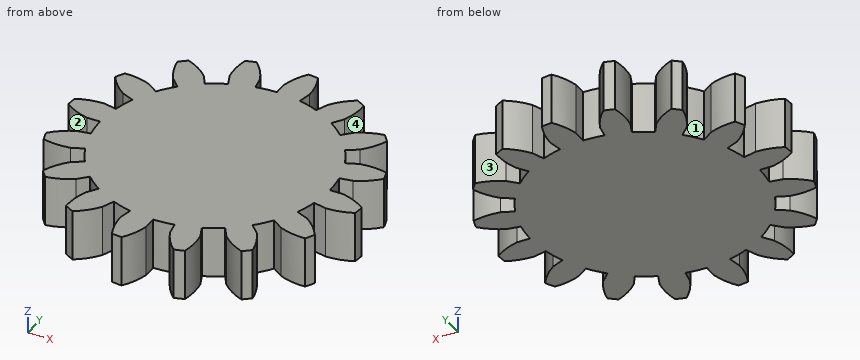
from build123d import *

# Parameters (mm, degrees)
BOSS_EXTRU_1_DEPTH           = 3
R_P_TITION_CIRCULAIRE2_COUNT = 16
ESQUISSE5_R                  = 6.75
BOSS_EXTRU_2_DEPTH           = 3


with BuildPart() as part:
    # Esquisse4 → Boss.-Extru.1 (new body)
    with BuildSketch(Plane.XY):
        with BuildLine():
            Line((0, 7.517540966), (0, 6.75))
            ThreePointArc((0, 6.75), (0.719454333, 6.711548664), (1.430711931, 6.59663273))
            Line((1.430711931, 6.59663273), (1.593397859, 7.346734339))
            ThreePointArc((1.593397859, 7.346734339), (1.508511555, 8.147299885), (1.256427196, 8.911867969))
            ThreePointArc((1.256427196, 8.911867969), (0.959272444, 8.948731551), (0.661055861, 8.975689675))
            ThreePointArc((0.661055861, 8.975689675), (0.252643326, 8.281924527), (0, 7.517540966))
        make_face()
    extrude(amount=BOSS_EXTRU_1_DEPTH)


with BuildPart() as r_p_tition_circulaire2_1:
    # R_p_tition circulaire2: pattern copy
    add(part.part.rotate(Axis((0, 0, 0), (0, 0, 1)), 1 * 360 / R_P_TITION_CIRCULAIRE2_COUNT))


with BuildPart() as r_p_tition_circulaire2_2:
    # R_p_tition circulaire2: pattern copy
    add(part.part.rotate(Axis((0, 0, 0), (0, 0, 1)), 2 * 360 / R_P_TITION_CIRCULAIRE2_COUNT))


with BuildPart() as r_p_tition_circulaire2_3:
    # R_p_tition circulaire2: pattern copy
    add(part.part.rotate(Axis((0, 0, 0), (0, 0, 1)), 3 * 360 / R_P_TITION_CIRCULAIRE2_COUNT))


with BuildPart() as r_p_tition_circulaire2_4:
    # R_p_tition circulaire2: pattern copy
    add(part.part.rotate(Axis((0, 0, 0), (0, 0, 1)), 4 * 360 / R_P_TITION_CIRCULAIRE2_COUNT))


with BuildPart() as r_p_tition_circulaire2_5:
    # R_p_tition circulaire2: pattern copy
    add(part.part.rotate(Axis((0, 0, 0), (0, 0, 1)), 5 * 360 / R_P_TITION_CIRCULAIRE2_COUNT))


with BuildPart() as r_p_tition_circulaire2_6:
    # R_p_tition circulaire2: pattern copy
    add(part.part.rotate(Axis((0, 0, 0), (0, 0, 1)), 6 * 360 / R_P_TITION_CIRCULAIRE2_COUNT))


with BuildPart() as r_p_tition_circulaire2_7:
    # R_p_tition circulaire2: pattern copy
    add(part.part.rotate(Axis((0, 0, 0), (0, 0, 1)), 7 * 360 / R_P_TITION_CIRCULAIRE2_COUNT))


with BuildPart() as r_p_tition_circulaire2_8:
    # R_p_tition circulaire2: pattern copy
    add(part.part.rotate(Axis((0, 0, 0), (0, 0, 1)), 8 * 360 / R_P_TITION_CIRCULAIRE2_COUNT))


with BuildPart() as r_p_tition_circulaire2_9:
    # R_p_tition circulaire2: pattern copy
    add(part.part.rotate(Axis((0, 0, 0), (0, 0, 1)), 9 * 360 / R_P_TITION_CIRCULAIRE2_COUNT))


with BuildPart() as r_p_tition_circulaire2_10:
    # R_p_tition circulaire2: pattern copy
    add(part.part.rotate(Axis((0, 0, 0), (0, 0, 1)), 10 * 360 / R_P_TITION_CIRCULAIRE2_COUNT))


with BuildPart() as r_p_tition_circulaire2_11:
    # R_p_tition circulaire2: pattern copy
    add(part.part.rotate(Axis((0, 0, 0), (0, 0, 1)), 11 * 360 / R_P_TITION_CIRCULAIRE2_COUNT))


with BuildPart() as r_p_tition_circulaire2_12:
    # R_p_tition circulaire2: pattern copy
    add(part.part.rotate(Axis((0, 0, 0), (0, 0, 1)), 12 * 360 / R_P_TITION_CIRCULAIRE2_COUNT))


with BuildPart() as r_p_tition_circulaire2_13:
    # R_p_tition circulaire2: pattern copy
    add(part.part.rotate(Axis((0, 0, 0), (0, 0, 1)), 13 * 360 / R_P_TITION_CIRCULAIRE2_COUNT))


with BuildPart() as r_p_tition_circulaire2_14:
    # R_p_tition circulaire2: pattern copy
    add(part.part.rotate(Axis((0, 0, 0), (0, 0, 1)), 14 * 360 / R_P_TITION_CIRCULAIRE2_COUNT))


with BuildPart() as r_p_tition_circulaire2_15:
    # R_p_tition circulaire2: pattern copy
    add(part.part.rotate(Axis((0, 0, 0), (0, 0, 1)), 15 * 360 / R_P_TITION_CIRCULAIRE2_COUNT))


with BuildPart() as part_1:
    add(part.part)

    add(r_p_tition_circulaire2_1.part)  # Boss.-Extru.2 merges R_p_tition circulaire2_1

    add(r_p_tition_circulaire2_2.part)  # Boss.-Extru.2 merges R_p_tition circulaire2_2

    add(r_p_tition_circulaire2_3.part)  # Boss.-Extru.2 merges R_p_tition circulaire2_3

    add(r_p_tition_circulaire2_4.part)  # Boss.-Extru.2 merges R_p_tition circulaire2_4

    add(r_p_tition_circulaire2_5.part)  # Boss.-Extru.2 merges R_p_tition circulaire2_5

    add(r_p_tition_circulaire2_6.part)  # Boss.-Extru.2 merges R_p_tition circulaire2_6

    add(r_p_tition_circulaire2_7.part)  # Boss.-Extru.2 merges R_p_tition circulaire2_7

    add(r_p_tition_circulaire2_8.part)  # Boss.-Extru.2 merges R_p_tition circulaire2_8

    add(r_p_tition_circulaire2_9.part)  # Boss.-Extru.2 merges R_p_tition circulaire2_9

    add(r_p_tition_circulaire2_10.part)  # Boss.-Extru.2 merges R_p_tition circulaire2_10

    add(r_p_tition_circulaire2_11.part)  # Boss.-Extru.2 merges R_p_tition circulaire2_11

    add(r_p_tition_circulaire2_12.part)  # Boss.-Extru.2 merges R_p_tition circulaire2_12

    add(r_p_tition_circulaire2_13.part)  # Boss.-Extru.2 merges R_p_tition circulaire2_13

    add(r_p_tition_circulaire2_14.part)  # Boss.-Extru.2 merges R_p_tition circulaire2_14

    add(r_p_tition_circulaire2_15.part)  # Boss.-Extru.2 merges R_p_tition circulaire2_15
    # Esquisse5 → Boss.-Extru.2 (add)
    with BuildSketch(Plane.XY):
        Circle(ESQUISSE5_R)
    extrude(amount=BOSS_EXTRU_2_DEPTH)


solid = part_1.part
Could you check a few things on this model? Use its own coordinates, in mm. Face numbers are marked on the shaded views. A direction names the side the tool comes from. Give positions to 0.01 mm unless a question says otherwise; leave off trailing zeros. Write each loop counter-clockwise with the first axis right and the second up, starting at its lowest first coordinate (ties: lowest second). Pieces come first, ordered by that corner, then holes. Notation, with made-up numbers: (-23, -6) -> (-11, -6) arc R24 cw to (-11, 4) -> close; hole circle Ø11 at (85.25, 17.25). An arc over 180 degrees is marked (long way). Answer as a JSON object with one key per item and string values.
Q1. Suppose I cut it at A-A on y = 3.25. Write out the boundary of the cut face in (x, z).
Taken from the geometry:
{"outline": "(-7.4, 0) -> (5.92, 0) -> (5.92, 3) -> (-7.4, 3) -> close"}
Q2. Which directions (+Z, -Z, +X, -X, +Y, -Y) give clear straight access to the entire face, cutting with the end or side of a thin tool? Please do the marked faces 1, 2, 3 and 4.
Taken from the geometry:
{"face 1": "+Z, -Z", "face 2": "+Z, -Z, -X", "face 3": "+Z, -Z, +Y", "face 4": "+Z, -Z, +X"}
Q3. Will these pins go through, and if not, where does the flat tip stop? pin 1 Ø2 at (x, y) = (7, 7) entering from +Z; pin 2 Ø0.8 at (y, z) = (-7, 1) entering from +X; pin 3 Ø1 at (y, z) = (-4, 2) entering from +X.
Taken from the geometry:
{"pin 1": "passes through", "pin 2": "stops at x = 5.88", "pin 3": "stops at x = 8.04"}
Q4. Please list where these lines run through material, in increasing order: L1, parallel to X at y = 7, z = 0.45; L2, parallel to X at y = 5, z = 0.9; L3, parallel to Y at x = 7.5, z = 1.3.
Taken from the geometry:
{"L1": "x = -5.66 to -4.99, -2.89 to -1.27, 0 to 1.52, 2.92 to 4.52", "L2": "x = -5 to 4.53, 5 to 7.01", "L3": "y = -4.57 to -3.35, -1.59 to 0, 1.38 to 2.94"}
